Autodesk Inventor part; units mm, degrees
ref_plane "YZ Plane" through (0, 0, 0) normal (1, 0, 0) x (0, 1, 0)
ref_plane "XZ Plane" through (0, 0, 0) normal (0, 1, 0) x (-1, 0, 0)
ref_plane "XY Plane" through (0, 0, 0) normal (0, 0, 1) x (1, 0, 0)
sketch "Sketch1" plane through (0, 0, 0) normal (0, 0, 1) x (1, 0, 0)
  line L0 (-36.75, 43) -> (36.75, 43)
  line L1 (36.75, 43) -> (36.75, -43)
  line L2 (36.75, -43) -> (-36.75, -43)
  line L3 (-36.75, -43) -> (-36.75, 43)
  point P0 (0, 0)
  point P1 (0, 43)
  point P2 (-36.75, 0)
  dimension "d0" = 73.5
  dimension "d1" = 86
extrude "Extrusion1" add sketch "Sketch1" along normal blind 8
sketch "Sketch4" plane through (0, 0, 0) normal (0, 0, -1) x (-1, 0, 0)
  line L0 (-36.75, -33) -> (-16.75, -33)
  line L1 (-16.75, -33) -> (-16.75, 33)
  line L2 (-16.75, 33) -> (-36.75, 33)
  line L3 (-36.75, 33) -> (-36.75, -33)
  line L4 (-36.75, -43) -> (-36.75, 43)
  point P0 (0, 0)
  point P1 (-36.75, 0)
  dimension "d19" = 20
  dimension "d20" = 66
extrude "Extrusion4" cut sketch "Sketch4" against normal blind 10
sketch "Sketch5" plane through (0, 0, 0) normal (0, 0, -1) x (-1, 0, 0)
  circle A0 centre (0.75, -24) radius 6
  circle A1 centre (0.75, 24) radius 6
  line L0 (-8.75, -33) -> (-8.75, 33)
  line L1 (-36.75, 33) -> (-36.75, 43)
  line L2 (-36.75, 43) -> (36.75, 43)
  line L3 (36.75, -43) -> (-36.75, -43)
  dimension "d23" = 12
  dimension "d37" = 37.5
  dimension "d38" = 19
  dimension "d39" = 19
extrude "Extrusion5" cut sketch "Sketch5" against normal blind 10
sketch "Sketch6" plane through (0, 0, 0) normal (0, 0, -1) x (-1, 0, 0)
  circle A0 centre (12.9988, 0) radius 11
  circle A1 centre (12.9988, -8) radius 1.75
  circle A2 centre (4.9988, 0) radius 1.75
  circle A3 centre (12.9988, 8) radius 1.75
  circle A4 centre (20.9988, 0) radius 1.75
  circle A5 centre (12.9988, 0) radius 5.5
  circle A6 centre (12.9988, 0) radius 8 construction
  line L0 (36.75, 43) -> (36.75, -43) construction
  line L1 (-36.75, 43) -> (36.75, 43) construction
  point P0 (0, 0)
  dimension "d42" = 3.5
  dimension "d43" = 11
  dimension "d44" = 23.7512
  dimension "d46" = 22
  dimension "d47" = 16
extrude "Extrusion6" cut sketch "Sketch6" against normal blind 10 contours A1 | A2 | A3 | A4 | A5
sketch "Sketch7" plane through (-36.75, 43, 0) normal (0, 1, 0) x (1, 0, 0)
  line L0 (73.5, 0) -> (73.5, -8)
  point P0 (36.75, 0)
  point P1 (58.5, -4)
  point P2 (67.5, -4)
  point P3 (73.5, -4)
  dimension "d48" = 9
  dimension "d49" = 6
hole "Hole1" at (21.75, 43, 4) at (30.75, 43, 4) direction (0, -1, 0) diameter 3.5 end through all
sketch "Sketch8" plane through (0, 0, 0) normal (0, 0, -1) x (-1, 0, 0)
  circle A0 centre (-16.75, 31.5) radius 1.5
  circle A1 centre (-16.75, -31.5) radius 1.5
  line L0 (-16.75, 33) -> (-16.75, -33)
  line L1 (-36.75, 33) -> (-16.75, 33)
  line L2 (-16.75, -33) -> (-36.75, -33)
  point P0 (0, 0)
  point P1 (-16.75, -30)
  point P2 (-16.75, 30)
  dimension "d57" = 3
  dimension "d58" = 3
extrude "Extrusion7" cut sketch "Sketch8" against normal through all contours A0 L0 | A1 L0 picked at (-15.9713, 31.7539) picked at (-16.4218, -31.037)
equation "\"d39\" = d38"
properties part number "0005-10-010"
The model under review builds one solid part; all positions refer to its coordinate system, in mm. A direction names the side the tool comes from. Give positions to 0.01 mm unless a question says otherwise; leave off trailing zeros. Write each loop counter-clockwise with the first axis right and the second up, starting at its lowest first coordinate (ties: lowest second). Pieces come first, ordered by that corner, then holes. Notation, with made-up numbers: M 59.5,83.5 L 87.5,83.5 A6 ccw 87.5,91.5 Z; hole C 81.25,3 d10. An arc over 180 degrees is marked long. One line per question, with ' | ' between items. Start each with the question number.
Item 1: We need section D-D on y = -37. Write out the cut boundary in (x, z).
Item 2: We need section A-A on z = 4. Give the number of separate pieces and of enclosed holes in the cut face, plus the area to 3 significant figures.
Item 3: Draft analysis for pull direction Z (two halves, no side actions). For faces 1 (the flat face through (-1, 1, 0)), 2 (the cylindrical face through (20, 38, 4)), 3 (the flat face through (16.75, 0, 4)), 4 (the cylindrical face through (20, -38, 4)), state which applies: released by +Z, released by -Z, zero draft, split by the parting line, or undercut.
Item 4: For faces 5 (the cylindrical face through (-3.25, 0.08, 3.94)), 6 (the flat face through (27, 33, 4)), list the 3-axis set-ups (+Z, -Z, +X, -X, +Y, -Y) from which the entire face can be reached by the end or side of a thin tool; tool diameter is ignored.
Item 5: We need section B-B on x = -0.75. Write out the cut boundary in (y, z), plus the area to 3 significant figures.
Item 6: For pin 1 (3 mm diameter, centred on x = -13, y = -8, fed in from -Z); pin 2 (10 mm diameter, centred on x = -1.5, y = -7, fed in from -Z), all flat-tipped, find the tip position at first contact; note any pin that passes through.
Item 7: Wall thickness on line 1 (X direction, y = -35.5, z = 4); line 2 (Y direction, x = 24, z = 3.75); line 3 (Y direction, x = 3.5, z = 4.5): over which ranges is each line inside the solid? List them lowest first. Write a range as from..to.
Item 8: We need section C-C on y = 24. Write out the cut boundary in (x, z), plus the area to 3 significant figures.
Results found:
1) outline: M -36.75,0 L 36.75,0 L 36.75,8 L -36.75,8 Z; hole C 21.75,4 d3.5; hole C 30.75,4 d3.5
2) separate pieces: 5 | enclosed holes: 7 | area: 4,490 mm2
3) face 1: released by -Z | face 2: undercut | face 3: zero draft | face 4: undercut
4) face 5: +Z, -Z | face 6: +Z, -Z, +X
5) outline: M -43,0 L -30,0 L -30,8 L -43,8 Z; M -18,0 L 18,0 L 18,8 L -18,8 Z; M 30,0 L 43,0 L 43,8 L 30,8 Z | area: 496 mm2
6) pin 1: passes through | pin 2: stops at z = 0
7) line 1: x = -36.75..20, 23.5..29, 32.5..36.75 | line 2: y = -43..-33, 33..43 | line 3: y = -43..-28.24, -19.76..19.76, 28.24..43
8) outline: M -36.75,0 L -6.75,0 L -6.75,8 L -36.75,8 Z; M 5.25,0 L 16.75,0 L 16.75,8 L 5.25,8 Z | area: 332 mm2
